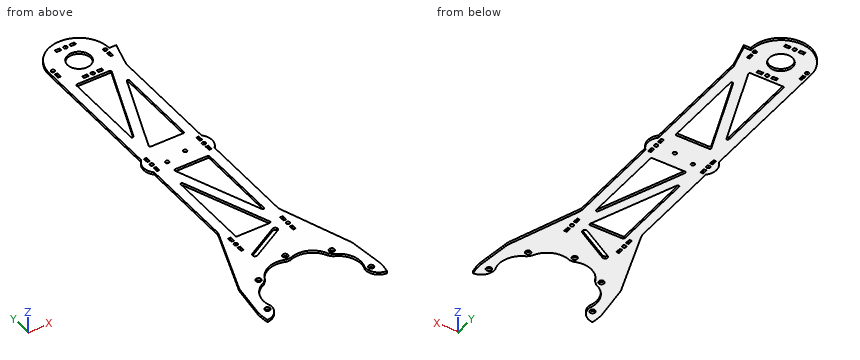
```python
from build123d import *

# Parameters (mm, degrees)
SKETCH_1_R      = 2.2
SKETCH_1_R_2    = 9.5
SKETCH_1_R_3    = 1.5
SKETCH_1_W      = 4.2
SKETCH_1_H      = 2.2
SKETCH_1_W_2    = 2.2
SKETCH_1_H_2    = 4.2
EXTRUDE_1_DEPTH = 2


with BuildPart() as part:
    # 草图1 → 凸台-拉伸1 (new body)
    with BuildSketch(Plane.XY):
        with BuildLine():
            Line((46.461426923, -96.447469622), (50, -125))
            ThreePointArc((50, -125), (49.748623245, -130.007441937), (48.997020592, -134.964533673))
            ThreePointArc((48.997020592, -134.964533673), (41.359915291, -131.321748354), (38.465512908, -123.370792619))
            ThreePointArc((38.465512908, -123.370792619), (38.545793672, -109.14087841), (28.474561687, -99.087660532))
            ThreePointArc((28.474561687, -99.087660532), (27.223611076, -97.776388924), (25.912339468, -96.525438313))
            ThreePointArc((25.912339468, -96.525438313), (15.85912159, -86.454206328), (1.629207381, -86.534487092))
            ThreePointArc((1.629207381, -86.534487092), (0, -86.5), (-1.629207381, -86.534487092))
            ThreePointArc((-1.629207381, -86.534487092), (-15.85912159, -86.454206328), (-25.912339468, -96.525438313))
            ThreePointArc((-25.912339468, -96.525438313), (-27.223611076, -97.776388924), (-28.474561687, -99.087660532))
            ThreePointArc((-28.474561687, -99.087660532), (-38.545793672, -109.14087841), (-38.465512908, -123.370792619))
            ThreePointArc((-38.465512908, -123.370792619), (-41.359915692, -131.321748192), (-48.997021107, -134.964533236))
            ThreePointArc((-48.997021107, -134.964533236), (-49.748623375, -130.007441694), (-50, -125))
            Line((-50, -125), (-46.461426923, -96.447469622))
            ThreePointArc((-46.461426923, -96.447469622), (-46.109594707, -94.783919835), (-45.481011279, -93.204025321))
            Line((-45.481011279, -93.204025321), (-25.348989293, -38.09742115))
            ThreePointArc((-25.348989293, -38.09742115), (-24.894773191, -36.408340658), (-24.741807932, -34.665955281))
            Line((-24.741807932, -34.665955281), (-24.741807932, -20.235407124))
            Line((-24.741807932, -20.235407124), (-24.741807932, 0))
            Line((-24.741807932, 0), (-24.741807932, 43.564592876))
            ThreePointArc((-24.741807932, 43.564592876), (-28.096937788, 51.664592876), (-24.741807932, 59.764592876))
            Line((-24.741807932, 59.764592876), (-24.741807932, 174.996783477))
            ThreePointArc((-24.741807932, 174.996783477), (0, 199.73859141), (24.741807932, 174.996783477))
            Line((24.741807932, 174.996783477), (30.452369558, 174.996783477))
            Line((30.452369558, 174.996783477), (24.741807932, 153.730120274))
            Line((24.741807932, 153.730120274), (24.741807932, 66.020820772))
            Line((24.741807932, 66.020820772), (24.741807932, 59.764592876))
            ThreePointArc((24.741807932, 59.764592876), (28.096937788, 51.664592876), (24.741807932, 43.564592876))
            Line((24.741807932, 43.564592876), (24.741807932, 37.305457961))
            Line((24.741807932, 37.305457961), (24.741807932, 0))
            Line((24.741807932, 0), (24.741807932, -20.235407124))
            Line((24.741807932, -20.235407124), (24.741807932, -34.665955281))
            ThreePointArc((24.741807932, -34.665955281), (24.894773191, -36.408340658), (25.348989293, -38.09742115))
            Line((25.348989293, -38.09742115), (45.481011279, -93.204025321))
            ThreePointArc((45.481011279, -93.204025321), (46.109594707, -94.783919835), (46.461426923, -96.447469622))
        make_face()
        with Locations((-42.5, -125)):
            Circle(SKETCH_1_R, mode=Mode.SUBTRACT)
        with Locations((-30.0520382, -94.9479618)):
            Circle(SKETCH_1_R, mode=Mode.SUBTRACT)
        with Locations((0, -82.5)):
            Circle(SKETCH_1_R, mode=Mode.SUBTRACT)
        with Locations((30.0520382, -94.9479618)):
            Circle(SKETCH_1_R, mode=Mode.SUBTRACT)
        with Locations((42.5, -125)):
            Circle(SKETCH_1_R, mode=Mode.SUBTRACT)
        with Locations((2.09e-07, 174.996783477)):
            Circle(SKETCH_1_R_2, mode=Mode.SUBTRACT)
        with Locations((0, 192.120903966)):
            Circle(SKETCH_1_R_3, mode=Mode.SUBTRACT)
        with Locations(Location((0, 157.879096034, 0), (0, 0, 180))):
            Circle(SKETCH_1_R_3, mode=Mode.SUBTRACT)
        with Locations((-21.392054648, -53.335407124)):
            Circle(SKETCH_1_R_3, mode=Mode.SUBTRACT)
        with Locations((-21.392054648, 51.664592876)):
            Circle(SKETCH_1_R_3, mode=Mode.SUBTRACT)
        with Locations(Location((21.392054648, -53.335407124, 0), (0, 0, 180))):
            Circle(SKETCH_1_R_3, mode=Mode.SUBTRACT)
        with Locations(Location((21.392054648, 51.664592876, 0), (0, 0, 180))):
            Circle(SKETCH_1_R_3, mode=Mode.SUBTRACT)
        with Locations(Location((21.447993697, 175, 0), (0, 0, 180))):
            Circle(SKETCH_1_R_3, mode=Mode.SUBTRACT)
        with Locations((-21.447993697, 175)):
            Circle(SKETCH_1_R_3, mode=Mode.SUBTRACT)
        with Locations((-10.976092936, 48.238908927)):
            Circle(SKETCH_1_R_3, mode=Mode.SUBTRACT)
        with Locations((6, 51.664592876)):
            Circle(SKETCH_1_R_3, mode=Mode.SUBTRACT)
        with Locations((6, 192.120903966)):
            Rectangle(SKETCH_1_W, SKETCH_1_H, mode=Mode.SUBTRACT)
        with Locations((-6, 192.120903966)):
            Rectangle(SKETCH_1_W, SKETCH_1_H, mode=Mode.SUBTRACT)
        with Locations((21.392054648, -47.335407124)):
            Rectangle(SKETCH_1_W_2, SKETCH_1_H_2, mode=Mode.SUBTRACT)
        with Locations((21.392054648, 45.664592876)):
            Rectangle(SKETCH_1_W_2, SKETCH_1_H_2, mode=Mode.SUBTRACT)
        with Locations((-21.447993697, 57.664592876)):
            Rectangle(SKETCH_1_W_2, SKETCH_1_H_2, mode=Mode.SUBTRACT)
        with Locations((-6, 157.879096034)):
            Rectangle(SKETCH_1_W, SKETCH_1_H, mode=Mode.SUBTRACT)
        with Locations((6, 157.879096034)):
            Rectangle(SKETCH_1_W, SKETCH_1_H, mode=Mode.SUBTRACT)
        with Locations((-21.392054648, -47.335407124)):
            Rectangle(SKETCH_1_W_2, SKETCH_1_H_2, mode=Mode.SUBTRACT)
        with Locations((-21.392054648, -59.335407124)):
            Rectangle(SKETCH_1_W_2, SKETCH_1_H_2, mode=Mode.SUBTRACT)
        with Locations((-21.392054648, 45.664592876)):
            Rectangle(SKETCH_1_W_2, SKETCH_1_H_2, mode=Mode.SUBTRACT)
        with BuildLine():
            Line((11.056492434, -56.33298533), (-15.666877498, -71.761730154))
            ThreePointArc((-15.666877498, -71.761730154), (-18.398928306, -71.029679346), (-17.666877498, -68.297628539))
            Line((-17.666877498, -68.297628539), (9.056492434, -52.868883715))
            ThreePointArc((9.056492434, -52.868883715), (11.788543242, -53.600934522), (11.056492434, -56.33298533))
        make_face(mode=Mode.SUBTRACT)
        with Locations((21.392054648, -59.335407124)):
            Rectangle(SKETCH_1_W_2, SKETCH_1_H_2, mode=Mode.SUBTRACT)
        with Locations((21.447993697, 57.664592876)):
            Rectangle(SKETCH_1_W_2, SKETCH_1_H_2, mode=Mode.SUBTRACT)
        with Locations((21.447993697, 169)):
            Rectangle(SKETCH_1_W_2, SKETCH_1_H_2, mode=Mode.SUBTRACT)
        with Locations((-21.447993697, 169)):
            Rectangle(SKETCH_1_W_2, SKETCH_1_H_2, mode=Mode.SUBTRACT)
        with BuildLine():
            Line((-16.741807932, 22.356006795), (-16.741807932, -45.600934522))
            ThreePointArc((-16.741807932, -45.600934522), (-16.448914714, -46.308041303), (-15.741807932, -46.600934522))
            Line((-15.741807932, -46.600934522), (10.976092936, -46.600934522))
            ThreePointArc((10.976092936, -46.600934522), (11.802499596, -46.164008258), (11.906748707, -45.235038586))
            Line((11.906748707, -45.235038586), (-14.811152161, 22.721902731))
            ThreePointArc((-14.811152161, 22.721902731), (-15.928012429, 23.338517806), (-16.741807932, 22.356006795))
        make_face(mode=Mode.SUBTRACT)
        with BuildLine():
            Line((-10.976092936, 38.564592876), (15.741807932, 38.564592876))
            ThreePointArc((15.741807932, 38.564592876), (16.448914714, 38.271699657), (16.741807932, 37.564592876))
            Line((16.741807932, 37.564592876), (16.741807932, -30.392348442))
            ThreePointArc((16.741807932, -30.392348442), (15.928012429, -31.374859452), (14.811152161, -30.758244377))
            Line((14.811152161, -30.758244377), (-11.906748707, 37.19869694))
            ThreePointArc((-11.906748707, 37.19869694), (-11.802499596, 38.127666612), (-10.976092936, 38.564592876))
        make_face(mode=Mode.SUBTRACT)
        with BuildLine():
            Line((14.811152161, 137.887430129), (-11.906748707, 69.930488812))
            ThreePointArc((-11.906748707, 69.930488812), (-11.802499596, 69.00151914), (-10.976092936, 68.564592876))
            Line((-10.976092936, 68.564592876), (15.741807932, 68.564592876))
            ThreePointArc((15.741807932, 68.564592876), (16.448914714, 68.857486095), (16.741807932, 69.564592876))
            Line((16.741807932, 69.564592876), (16.741807932, 137.521534193))
            ThreePointArc((16.741807932, 137.521534193), (15.928012429, 138.504045204), (14.811152161, 137.887430129))
        make_face(mode=Mode.SUBTRACT)
        with BuildLine():
            Line((11.906748707, 152.364224338), (-14.811152161, 84.407283021))
            ThreePointArc((-14.811152161, 84.407283021), (-15.928012429, 83.790667946), (-16.741807932, 84.773178956))
            Line((-16.741807932, 84.773178956), (-16.741807932, 152.730120274))
            ThreePointArc((-16.741807932, 152.730120274), (-16.448914714, 153.437227055), (-15.741807932, 153.730120274))
            Line((-15.741807932, 153.730120274), (10.976092936, 153.730120274))
            ThreePointArc((10.976092936, 153.730120274), (11.802499596, 153.29319401), (11.906748707, 152.364224338))
        make_face(mode=Mode.SUBTRACT)
    extrude(amount=EXTRUDE_1_DEPTH)


solid = part.part
```
Input: part model. Units: mm. Frame: model coordinates. Round coordinates to 2 decimals unless told otherwise and drop trailing zeros. Order: outer loops, then holes, each group sorted by start corner. A loop starts at its lowest first (then second) coordinate and runs counter-clockwise, first axis right, second up. Notation, with made-up numbers: (67.25, -18.5) - (120.25, -18.5) arc R11 cw to (120.25, -14.5) - close; hole circle Ø6 at (64.25, 86.5). An arc over 180 degrees is marked (long way). One line per question, with ' | ' between items. Start each with the question number.
1) Contact query for flat-ended pins moving along their axis: P1, Ø1, axis at y = -60, z = 1, coming from the +X side; P2, Ø1, axis at x = 19.5, z = 0.5, coming from the -Y side; P3, Ø0.6, axis at y = 46.5, z = 1, coming from the +X side. Output: stop coordinate, or through.
2) Cut plane D-D, the plane x = -35.5. Return the cut outline in (y, z).
3) Cut plane A-A, the plane y = -65. Return the cut outline in (x, z), then the cut area to 3 significant figures.
4) Cut plane B-B, the plane y = -106.5. Return the cut outline in (x, z).
5) Ray query, probe 1 along X at (y, z) = (169, 0.25); probe 2 along X at (y, z) = (111, 1.15); probe 3 along X at (y, z) = (52, 1.15). Return the intervals inside material, ascending.
6) Cut plane C-C, the plane z = 0.3. Give the number of separate pieces and of enclosed holes in the cut face, then the cut area to 3 significant figures.
Worked out:
1) P1: stops at x = 33.53 | P2: stops at y = -88.83 | P3: stops at x = 27.01
2) outline: (-104.16, 0) - (-65.88, 0) - (-65.88, 2) - (-104.16, 2) - close
3) outline: (-35.18, 0) - (-11.96, 0) - (-11.96, 2) - (-35.18, 2) - close; (-3.96, 0) - (35.18, 0) - (35.18, 2) - (-3.96, 2) - close | area: 125 mm^2
4) outline: (-47.71, 0) - (-37.2, 0) - (-37.2, 2) - (-47.71, 2) - close; (37.2, 0) - (47.71, 0) - (47.71, 2) - (37.2, 2) - close
5) probe 1: x = -24.74 to -22.55, -20.35 to -7.37, 7.37 to 20.35, 22.55 to 28.84 | probe 2: x = -24.74 to -16.74, -4.36 to 4.24, 16.74 to 24.74 | probe 3: x = -28.09 to -22.85, -19.93 to 4.54, 7.46 to 19.93, 22.85 to 28.09
6) separate pieces: 1 | enclosed holes: 35 | area: 11,200 mm^2
